```python
from build123d import *

# Parameters (mm, degrees)
SKETCH1_W           = 63
SKETCH1_H           = 25
SKETCH1_R           = 3.8
BOSS_EXTRUDE1_DEPTH = 2
SKETCH1_3_R         = 2.05
BOSS_EXTRUDE2_DEPTH = 2


with BuildPart() as part:
    # Sketch1 → Boss-Extrude1 (new body)
    with BuildSketch(Plane.XY):
        with Locations((0, -2.5)):
            Rectangle(SKETCH1_W, SKETCH1_H)
        with Locations((-23, 4)):
            Circle(SKETCH1_R, mode=Mode.SUBTRACT)
        with Locations((-23, -9)):
            Circle(SKETCH1_R, mode=Mode.SUBTRACT)
        with Locations((23, -9)):
            Circle(SKETCH1_R, mode=Mode.SUBTRACT)
        with Locations((23, 4)):
            Circle(SKETCH1_R, mode=Mode.SUBTRACT)
    extrude(amount=BOSS_EXTRUDE1_DEPTH)

    # Sketch1_3 → Boss-Extrude2 (add)
    with BuildSketch(Plane.XY):
        Polygon((0, -37.51566868), (13, -37.51566868), (31.5, -15), (-31.5, -15), (-13, -37.51566868), align=None)
        with Locations((0, -31.299955557)):
            Circle(SKETCH1_3_R, mode=Mode.SUBTRACT)
        with Locations((0, -21.322069584)):
            Circle(SKETCH1_3_R, mode=Mode.SUBTRACT)
    extrude(amount=BOSS_EXTRUDE2_DEPTH)


solid = part.part
```
CAD build for the part. Positions are in the model's coordinates, mm. Round coordinates to 2 decimals unless told otherwise and drop trailing zeros. Loops run counter-clockwise (first coordinate to the right, second up) from the corner with the lowest first, then second, coordinate; pieces in that order, holes last. Notation, with made-up numbers: (43.25, -11.5) - (76.25, -11.5) arc R13 ccw to (76.25, 2.5) - close; hole circle Ø2 at (6.25, 36.5). An arc over 180 degrees is marked (long way). Return JSON: item names as keys, results as strings. Group by question number.
Q1. Band-saw the part on D-D on x = -18. Give the cut face in (y, z).
Q2. Flat gauge pins, fed straight in: pin 1 Ø10 at (x, y) = (-23, -9) entering from -Z; pin 2 Ø3.5 at (x, y) = (0, -21.32) entering from +Z; pin 3 Ø1 at (x, z) = (23.5, 0.5) entering from -Y; pin 4 Ø1 at (x, z) = (19.5, 1) entering from -Y. Where does each tip first touch, or does it go through?
Q3. Band-saw the part on C-C on z = 1.1. Give the cut face in (x, y), plus the area to 3 significant figures.
Q4. Two-plate mould, pull along X, no slides. Class faces 1 (the face through (22.12, -26.415, 0.986)), 2 (the face through (0, -13, 0)), 3 (the face through (-19.375, 5.141, 0.986)): +X half, -X half, draft (parallel to the pull), parting line (faces both ways), or undercut.
Q5. Band-saw the part on A-A on x = 0. Give the cut face in (y, z), plus the area to 3 significant figures.
Q6. Drill centre lines: line 1 along Y through (x, z) = (0, 1); line 2 along Y through (x, z) = (-23, 0.85); line 3 along X through (y, z) = (-7.5, 1.2). Where is each one in solid material? Low to high. Write a range as [from, to].
Q7. Band-saw the part on B-B on y = -9. Give the cut face in (x, z), plus the area to 3 significant figures.
Solutions:
{
 "1": {"outline": "(-31.43, 0) - (10, 0) - (10, 2) - (-31.43, 2) - close"},
 "2": {"pin 1": "stops at z = 0", "pin 2": "passes through", "pin 3": "stops at y = -25.35", "pin 4": "stops at y = -30.21"},
 "3": {"outline": "(-31.5, -15) - (-13, -37.52) - (13, -37.52) - (31.5, -15) - (31.5, 10) - (-31.5, 10) - close; hole circle Ø7.6 at (-23, -9); hole circle Ø7.6 at (-23, 4); hole circle Ø4.1 at (0, -31.3); hole circle Ø4.1 at (0, -21.32); hole circle Ø7.6 at (23, -9); hole circle Ø7.6 at (23, 4)", "area": "2,370 mm^2"},
 "4": {"face 1": "+X half", "face 2": "draft", "face 3": "undercut"},
 "5": {"outline": "(-37.52, 0) - (-33.35, 0) - (-33.35, 2) - (-37.52, 2) - close; (-29.25, 0) - (-23.37, 0) - (-23.37, 2) - (-29.25, 2) - close; (-19.27, 0) - (10, 0) - (10, 2) - (-19.27, 2) - close", "area": "78.6 mm^2"},
 "6": {"line 1": "y = [-37.52, -33.35], [-29.25, -23.37], [-19.27, 10]", "line 2": "y = [-25.35, -12.8], [-5.2, 0.2], [7.8, 10]", "line 3": "x = [-31.5, -26.49], [-19.51, 19.51], [26.49, 31.5]"},
 "7": {"outline": "(-31.5, 0) - (-26.8, 0) - (-26.8, 2) - (-31.5, 2) - close; (-19.2, 0) - (19.2, 0) - (19.2, 2) - (-19.2, 2) - close; (26.8, 0) - (31.5, 0) - (31.5, 2) - (26.8, 2) - close", "area": "95.6 mm^2"}
}
